from build123d import *

# Parameters (mm, degrees)
SKETCH1_R               = 6
BOSS_EXTRUDE1_DEPTH     = 106
CUT_EXTRUDE1_DEPTH      = 107.339080304
CUT_EXTRUDE1_DEPTH_BACK = 107.339080304
SKETCH2_R               = 1.5
CUT_EXTRUDE2_DEPTH      = 10
CHAMFER1_SIZE           = 0.5


with BuildPart() as part:
    # Sketch1 → Boss-Extrude1 (new body)
    with BuildSketch(Plane.XY):
        Circle(SKETCH1_R)
    extrude(amount=-BOSS_EXTRUDE1_DEPTH)

    # Sketch2 → Cut-Extrude1 (cut, two sides: drawn at the far end of the back side and taken through both)
    with BuildSketch(Plane(origin=(0, 0, 0), x_dir=(0, 0, -1), z_dir=(1, 0, 0)).offset(-CUT_EXTRUDE1_DEPTH_BACK)):
        with Locations(Location((101, 0, 0), (0, 0, 180))):
            Circle(SKETCH2_R)
    extrude(amount=CUT_EXTRUDE1_DEPTH + CUT_EXTRUDE1_DEPTH_BACK, mode=Mode.SUBTRACT)

    # Sketch3 → Cut-Extrude2 (cut)
    with BuildSketch(Plane.XY):
        with BuildLine():
            Line((-3.968626967, 4.5), (3.968626967, 4.5))
            ThreePointArc((3.968626967, 4.5), (0, 6), (-3.968626967, 4.5))
        make_face()
    extrude(amount=-CUT_EXTRUDE2_DEPTH, mode=Mode.SUBTRACT)

    # Chamfer1
    chamfer1_edges = [part.edges().sort_by_distance(p)[0] for p in [
        (-2.468626967, -5.468626967, 0),
        (0, 4.5, 0),
        (-6, 0, -106),
    ]]
    chamfer(chamfer1_edges, length=CHAMFER1_SIZE)


solid = part.part
CAD build for the part. Positions are in the model's coordinates, mm. A direction names the side the tool comes from. Round coordinates to 2 decimals unless told otherwise and drop trailing zeros. Write each loop counter-clockwise with the first axis right and the second up, starting at its lowest first coordinate (ties: lowest second). Pieces come first, ordered by that corner, then holes.
(1) 3-axis set-ups, long thin cutter, end or side, ignore diameter. For faces 1 (the face through (0, 4.5, -5)), 2 (the face through (0, -1, 0)): which of +Z, -Z, +X, -X, +Y, -Y reach the whole face in a straight line?
(2) Drop flat-ended pins along their axis: P1, Ø1, axis at x = 0.5, y = 2.5, coming from the +Z side; P2, Ø1.5, axis at x = -4, z = -25, coming from the -Y side; P3, Ø3, axis at y = 2.5, z = -92, coming from the +X side; P4, Ø3, axis at y = -3, z = -22.5, coming from the +X side. Give the stop position or say it passes through.
(3) Slice it at B-B, the plane z = -12. Write the cut outline in (x, y).
(4) Slice it at A-A, the plane x = 0. Write the cut outline in (y, z), and give its area (3 significant figures).
(5) Mould opens along Y. For faces 3 (the face through (-1.301, -5.857, -52.265)), 4 (the face through (-0.084, -1.265, -100.194)), 5 (the face through (0, 0, -106)) say: pulls with the +Y half, pulls with the -Y half, needs draft (parallel to the pull), parting line crosses it, or undercut.
(6) Probe line 1 along Z through (x, y) = (-5, -0.25); line 2 along Y through (x, z) = (0.25, -38.5); line 3 along X through (y, z) = (-0.5, -85.5). List the from-to ranges inside material, lowest first.
(7) Slice it at C-C, the plane z = -101. Write the cut outline in (x, y), and give its area (3 significant figures).
From the geometry:
1. face 1: +Z, +X, -X, +Y
1. face 2: +Z, +X, -X, +Y, -Y
2. P1: stops at z = 0
2. P2: stops at y = -5.04
2. P3: stops at x = 5.92
2. P4: stops at x = 5.81
3. outline: circle Ø12 at (0, 0)
4. outline: (-6, -105.5) - (-5.5, -106) - (5.5, -106) - (6, -105.5) - (6, -10) - (4.5, -10) - (4.5, -0.5) - (4, 0) - (-5.5, 0) - (-6, -0.5) - close; hole circle Ø3 at (0, -101)
4. area: 1,250 mm2
5. face 3: parting line crosses it
5. face 4: undercut
5. face 5: needs draft
6. line 1: z = -106 to -102.48, -99.52 to 0
6. line 2: y = -5.99 to 5.99
6. line 3: x = -5.98 to 5.98
7. outline: (-5.81, -1.5) arc R6 ccw to (5.81, -1.5) - close; (-5.81, 1.5) - (5.81, 1.5) arc R6 ccw to start
7. area: 77.5 mm2
